from build123d import *

# Parameters (mm, degrees)
SALIENTE_EXTRUIR1_DEPTH = 10
CROQUIS2_R              = 2
CORTAR_EXTRUIR2_DEPTH   = 30
CORTAR_EXTRUIR3_START   = -10
CORTAR_EXTRUIR3_DEPTH   = 10


with BuildPart() as part:
    # Croquis1 → Saliente-Extruir1 (new body)
    with BuildSketch(Plane.XY):
        with BuildLine():
            Line((2, 0), (8, 0))
            ThreePointArc((8, 0), (9.414213562, 0.585786438), (10, 2))
            Line((10, 2), (10, 22))
            ThreePointArc((10, 22), (12.343145751, 27.656854249), (18, 30))
            Line((18, 30), (36, 30))
            ThreePointArc((36, 30), (38.828427125, 31.171572875), (40, 34))
            Line((40, 34), (40, 36))
            ThreePointArc((40, 36), (38.828427125, 38.828427125), (36, 40))
            Line((36, 40), (8, 40))
            ThreePointArc((8, 40), (2.343145751, 37.656854249), (0, 32))
            Line((0, 32), (0, 2))
            ThreePointArc((0, 2), (0.585786438, 0.585786438), (2, 0))
        make_face()
    extrude(amount=SALIENTE_EXTRUIR1_DEPTH)

    # Croquis2 → Cortar-Extruir2 (cut)
    with BuildSketch(Plane(origin=(0, 40, 0), x_dir=(1, 0, 0), z_dir=(0, 1, 0))):
        with Locations(Location((16.696699141, -5.303300859, 0), (0, 0, 180))):
            Circle(CROQUIS2_R)
        with Locations(Location((27.303300859, -5.303300859, 0), (0, 0, 180))):
            Circle(CROQUIS2_R)
    extrude(amount=-CORTAR_EXTRUIR2_DEPTH, mode=Mode.SUBTRACT)

    # Croquis3 → Cortar-Extruir3 (cut)
    with BuildSketch(Plane.XY.offset(10).offset(CORTAR_EXTRUIR3_START)):
        with BuildLine():
            Line((32, 36.83772234), (32, 33.16227766))
            ThreePointArc((32, 33.16227766), (31.458039892, 31.291448967), (30, 30))
            Line((30, 30), (36, 30))
            ThreePointArc((36, 30), (38.828427125, 31.171572875), (40, 34))
            Line((40, 34), (40, 36))
            ThreePointArc((40, 36), (38.828427125, 38.828427125), (36, 40))
            Line((36, 40), (30, 40))
            ThreePointArc((30, 40), (31.458039892, 38.708551033), (32, 36.83772234))
        make_face()
    extrude(amount=CORTAR_EXTRUIR3_DEPTH, mode=Mode.SUBTRACT)


solid = part.part
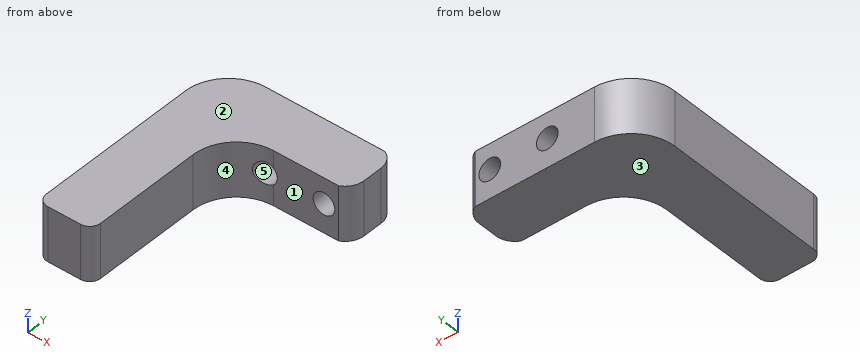
Source: CAD feature listing. Evaluate the final solid. Frame: model axes, mm. Face numbers are marked on the shaded views. A direction names the side the tool comes from. Give positions to 0.01 mm unless a question says otherwise; leave off trailing zeros. Write each loop counter-clockwise with the first axis right and the second up, starting at its lowest first coordinate (ties: lowest second). Pieces come first, ordered by that corner, then holes. Notation, with made-up numbers: (57, 14) -> (70, 14) arc R20 ccw to (70, 46) -> close; hole circle Ø11 at (-31.75, 12). An arc over 180 degrees is marked (long way). Write item = value, one per line.
Q1. Mould query, pull axis X, two halves, no side actions, for the marked faces 3, 4 and 5. Classes: +X half, -X half, draft (parallel to the pull), parting line (faces both ways), or undercut.
Here are the results:
face_3 = draft
face_4 = +X half
face_5 = undercut
Q2. Cut plane D-D on y = 9.5. Return loops of the section in (x, z), then the cut area to 3 significant figures.
Here are the results:
outline = (0, 0) -> (10, 0) -> (10, 10) -> (0, 10) -> close
area = 100 mm²
Q3. Line query: line 1 (Z direction, x = 27.5, y = 30.5); line 2 (X direction, y = 16, z = 7.5); line 3 (X direction, y = 33.5, z = 5.75). Output: solid intervals per line, ascending. Write a range as from..to.
Here are the results:
line_1 = 0..3.31, 7.29..10
line_2 = 0..10
line_3 = 0.14..14.75, 18.65..25.35, 29.25..32
Q4. Cut plane A-A on z = 9.25. Return loops of the section in (x, y).
Here are the results:
outline = (0, 2) arc R2 ccw to (2, 0) -> (8, 0) arc R2 ccw to (10, 2) -> (10, 22) arc R8 cw to (18, 30) -> (30, 30) arc R3.5 ccw to (32, 33.16) -> (32, 36.84) arc R3.5 ccw to (30, 40) -> (8, 40) arc R8 ccw to (0, 32) -> close
Q5. Reachability of the marked faces 1 and 2 from +Z, -Z, +X, -X, +Y, -Y: full face, straight path, thin tool, end or side. Return the list, or none.
Here are the results:
face_1 = +Z, -Z, +X, -Y
face_2 = +Z, +X, -X, +Y, -Y
Q6. First-contact query: pin 1 (3 mm diameter, centred on x = 25, z = 7, fed in from -Y); pin 2 (4 mm diameter, centred on y = 4, z = 8, fed in from +X); pin 3 (5 mm diameter, centred on x = 16.7, z = 5.3, fed in from -Y); pin 4 (8 mm diameter, centred on x = 15, y = 8.5, fed in from -Z). Flat tips, straight axial feed; report the tip coordinate or a pass-through.
Here are the results:
pin_1 = 30
pin_2 = 10
pin_3 = 29.04
pin_4 = through
Q7. Cut plane B-B on z = 4.5. Return loops of the section in (x, y), then the cut area to 3 significant figures.
Here are the results:
outline = (0, 2) arc R2 ccw to (2, 0) -> (8, 0) arc R2 ccw to (10, 2) -> (10, 22) arc R8 cw to (14.87, 29.36) -> (14.87, 40) -> (8, 40) arc R8 ccw to (0, 32) -> close; (18.53, 30) -> (25.47, 30) -> (25.47, 40) -> (18.53, 40) -> close; (29.13, 30) -> (30, 30) arc R3.5 ccw to (32, 33.16) -> (32, 36.84) arc R3.5 ccw to (30, 40) -> (29.13, 40) -> close
area = 541 mm²
Q8. Cut plane C-C on y = 37.5. Return loops of the section in (x, z), then the cut area to 3 significant figures.
Here are the results:
outline = (2.19, 0) -> (31.94, 0) -> (31.94, 10) -> (2.19, 10) -> close; hole circle Ø4 at (16.7, 5.3); hole circle Ø4 at (27.3, 5.3)
area = 272 mm²
